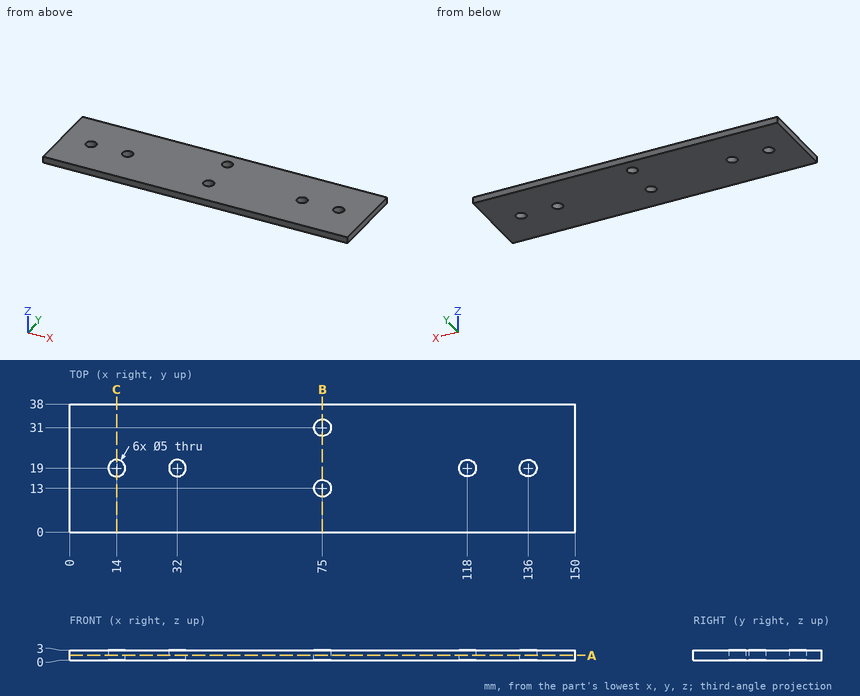
Answer from the drawing. Dimensions are ordinates in mm from the lowest x, y and z of the part. Coordinates: 2 decimals unless noted, no trailing zeros. Loops run counter-clockwise (first coordinate to the right, second up) from the corner with the lowest first, then second, coordinate; pieces in that order, holes last. Notation, with made-up numbers: (26.5, 67.5) - (39.5, 67.5) arc R4 ccw to (39.5, 72.5) - close; hole circle Ø3 at (61.25, 87.5). An arc over 180 degrees is marked (long way). Use a Markdown table: item, result.
Item 1: Find section C-C, the plane x = 14. Determine the outline of the cut face in (y, z).
Evaluation:
| item | result |
|---|---|
| outline | (0, 0) - (16.5, 0) - (16.5, 3) - (0, 3) - close; (21.5, 0) - (38, 0) - (38, 3) - (21.5, 3) - close |
Item 2: Find section A-A, the plane z = 1.45. Determine the outline of the cut face in (x, y).
Evaluation:
| item | result |
|---|---|
| outline | (0, 0) - (150, 0) - (150, 38) - (0, 38) - close; hole circle Ø5 at (14, 19); hole circle Ø5 at (32, 19); hole circle Ø5 at (75, 13); hole circle Ø5 at (75, 31); hole circle Ø5 at (118, 19); hole circle Ø5 at (136, 19) |
Item 3: Find section B-B, the plane x = 75. Determine the outline of the cut face in (y, z).
Evaluation:
| item | result |
|---|---|
| outline | (0, 0) - (10.5, 0) - (10.5, 3) - (0, 3) - close; (15.5, 0) - (28.5, 0) - (28.5, 3) - (15.5, 3) - close; (33.5, 0) - (38, 0) - (38, 3) - (33.5, 3) - close |
Item 4: Given pin 1 Ø3 at (x, y) = (75, 31) entering from +Z, flat-ended and moving along its own axis, determine where the tip first touches the part or whether it passes through.
Evaluation:
| item | result |
|---|---|
| pin 1 | passes through |
Item 5: Consider probe 1 along Y at (x, z) = (136, 1.45); probe 2 along X at (y, z) = (12.5, 0.4); probe 3 along Y at (x, z) = (138, 1.25). Determine where each line is inside the solid, lowest interval first. Write a range as from..to.
Evaluation:
| item | result |
|---|---|
| probe 1 | y = 0..16.5, 21.5..38 |
| probe 2 | x = 0..72.55, 77.45..150 |
| probe 3 | y = 0..17.5, 20.5..38 |
